Part model, mm, in its own coordinate system. Face numbers are marked on the shaded views. Round coordinates to 2 decimals unless told otherwise and drop trailing zeros. Write each loop counter-clockwise with the first axis right and the second up, starting at its lowest first coordinate (ties: lowest second). Pieces come first, ordered by that corner, then holes. Notation, with made-up numbers: M 34.5,78.25 L 93.5,78.25 A18 cw 93.5,107.25 Z; hole C 48,-16.75 d3. An arc over 180 degrees is marked long. Use a Markdown table: item, result. Add a question column.
1) Two-plate mould, pull along Y, no slides. Class the marked faces 1 and 2: released by +Y, released by -Y, zero draft, split by the parting line, or undercut.
2) Drop flat-ended pins along their axis: P1, Ø3, axis at x = -81.61, y = 42.75, coming from the +Z side (3 decimals); P2, Ø1, axis at y = 17.5, z = 4, coming from the -X side; P3, Ø2.5, axis at x = -2, z = 5, coming from the -Y side; P4, Ø3.5, axis at y = 16, z = 5.5, coming from the +X side. Give the stop position or say it passes through.
3) Slice it at A-A on z = 4.75. Give the number of separate pieces and of enclosed holes in the cut face, plus the area to 3 significant figures.
4) Slice it at C-C on x = -56. Write the cut outline in (y, z) (3 decimals).
5) Wall check: probe 1 along X at (y, z) = (52.5, 4.5) (3 decimals); probe 2 along Y at (x, z) = (-3.5, 3.5) (3 decimals); probe 3 along X at (y, z) = (32, 4.25) (3 decimals). Give the ranges that are in metal, low to high.
6) Slice it at B-B on y = -5. Write the cut outline in (x, z) (3 decimals), plus the area to 3 significant figures.
7) Slice it at D-D on x = 53. Write the cut outline in (y, z) (3 decimals).
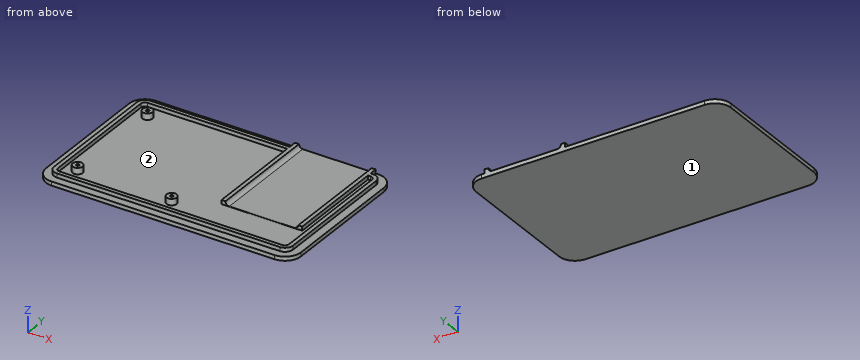
```python
from build123d import *

# Parameters (mm, degrees)
F0_W             = 203.2
F0_H             = 127
F1_DEPTH         = 3.175
F2_R             = 12.7
F4_DEPTH         = 3.175
F5_T             = -3.175
F6_W             = 58
F6_H             = 9.525
F7_DEPTH         = 3.176
F9_DEPTH         = 90
F10_DEPTH        = 3.175
F11_DEPTH        = 3.175
F12_R            = 4
F13_DEPTH        = 5
F17_D            = 2.5
F17_DEPTH        = 5
F17_TIP          = 0.7510757738
F17_ON_F15_D     = 2.5
F17_ON_F15_DEPTH = 5
F17_ON_F15_TIP   = 0.7510757738
F17_ON_F16_D     = 2.5
F17_ON_F16_DEPTH = 5
F17_ON_F16_TIP   = 0.7510757738


# Not quite as in the source:
# - a feature names something its author has since deleted; it is built from what else it names


with BuildPart() as f1:
    # F0 (on Top) → F1 (new body)
    with BuildSketch(Plane.XY):
        Rectangle(F0_W, F0_H)
    extrude(amount=F1_DEPTH)

    # F2
    f2_edges = [f1.edges().sort_by_distance(p)[0] for p in [
        (-101.6, -63.5, 1.5875),
        (-101.6, 63.5, 1.5875),
        (101.6, -63.5, 1.5875),
        (101.6, 63.5, 1.5875),
    ]]
    fillet(f2_edges, radius=F2_R)

    # F3 (on face) → F4 (join)
    with BuildSketch(Plane.XY.offset(3.175)):
        with BuildLine():
            Line((88.9, 57.15), (-88.9, 57.15))
            ThreePointArc((-88.9, 57.15), (-93.3901280605, 55.2901280605), (-95.25, 50.8))
            Line((-95.25, 50.8), (-95.25, -50.8))
            ThreePointArc((-95.25, -50.8), (-93.3901280605, -55.2901280605), (-88.9, -57.15))
            Line((-88.9, -57.15), (88.9, -57.15))
            ThreePointArc((88.9, -57.15), (93.3901280605, -55.2901280605), (95.25, -50.8))
            Line((95.25, -50.8), (95.25, 50.8))
            ThreePointArc((95.25, 50.8), (93.3901280605, 55.2901280605), (88.9, 57.15))
        make_face()
    extrude(amount=F4_DEPTH)

    # F5
    f5_openings = [f1.faces().sort_by_distance(p)[0] for p in [
        (0, 0, 6.35),
    ]]
    offset(amount=F5_T, openings=f5_openings, kind=Kind.INTERSECTION)

    # F6 (on face) → F7 (cut, through all)
    with BuildSketch(Plane.XY.offset(3.175)):
        with Locations((54.6, 58.7375)):
            Rectangle(F6_W, F6_H)
    extrude(amount=F7_DEPTH, mode=Mode.SUBTRACT)

    # F8 (on face) → F9 (join)
    with BuildSketch(Plane(origin=(0, 63.5, 0), x_dir=(-1, 0, 0), z_dir=(0, 1, 0))):
        with BuildLine():
            Line((-83.6, 6.35), (-83.6, 3.175))
            Line((-83.6, 3.175), (-25.6, 3.175))
            Line((-25.6, 3.175), (-25.6, 6.35))
            ThreePointArc((-25.6, 6.35), (-26.4786796564, 4.2286796564), (-28.6, 3.35))
            Line((-28.6, 3.35), (-80.6, 3.35))
            ThreePointArc((-80.6, 3.35), (-82.7213203436, 4.2286796564), (-83.6, 6.35))
        make_face()
    extrude(amount=-F9_DEPTH)

    # F10 (add): faces of the model
    f10_faces = [f1.faces().sort_by_distance(p)[0] for p in [
        (25.6, 13.7375, 4.7625),
        (25.6, 60.325, 4.7625),
    ]]
    extrude(f10_faces, amount=F10_DEPTH)

    # F11 (add): faces of the model
    f11_faces = [f1.faces().sort_by_distance(p)[0] for p in [
        (83.6, 13.7375, 4.7625),
        (83.6, 60.325, 4.7625),
    ]]
    extrude(f11_faces, amount=F11_DEPTH)

    # F12 (on face) → F13 (join)
    with BuildSketch(Plane.XY.offset(3.175)):
        with Locations((-81.6051200401, -42.75)):
            Circle(F12_R)
        with Locations((-6.7051200401, -42.75)):
            Circle(F12_R)
        with Locations((-81.6051200401, 42.75)):
            Circle(F12_R)
    extrude(amount=F13_DEPTH)

    # F17
    with Locations(Plane.XY.offset(8.175)):
        with Locations((-81.6051200401, 42.75)):
            Hole(F17_D / 2, depth=F17_DEPTH)
            with Locations((0, 0, -(F17_DEPTH + F17_TIP / 2))):  # 118° drill point
                Cone(0, F17_D / 2, F17_TIP, mode=Mode.SUBTRACT)

    # F17 on F15
    with Locations(Plane.XY.offset(8.175)):
        with Locations((-81.6051200401, -42.75)):
            Hole(F17_ON_F15_D / 2, depth=F17_ON_F15_DEPTH)
            with Locations((0, 0, -(F17_ON_F15_DEPTH + F17_ON_F15_TIP / 2))):  # 118° drill point
                Cone(0, F17_ON_F15_D / 2, F17_ON_F15_TIP, mode=Mode.SUBTRACT)

    # F17 on F16
    with Locations(Plane.XY.offset(8.175)):
        with Locations((-6.7051200401, -42.75)):
            Hole(F17_ON_F16_D / 2, depth=F17_ON_F16_DEPTH)
            with Locations((0, 0, -(F17_ON_F16_DEPTH + F17_ON_F16_TIP / 2))):  # 118° drill point
                Cone(0, F17_ON_F16_D / 2, F17_ON_F16_TIP, mode=Mode.SUBTRACT)


solid = f1.part
```
Entries:
| question | item | result |
|---|---|---|
| 1 | face 1 | zero draft |
| 1 | face 2 | undercut |
| 2 | P1 | stops at z = 8.175 |
| 2 | P2 | stops at x = -95.25 |
| 2 | P3 | stops at y = -57.15 |
| 2 | P4 | stops at x = 95.25 |
| 3 | separate pieces | 4 |
| 3 | enclosed holes | 3 |
| 3 | area | 2,460 mm^2 |
| 4 | outline | M -63.5,0 L 63.5,0 L 63.5,3.175 L 57.15,3.175 L 57.15,6.35 L 53.975,6.35 L 53.975,3.175 L -53.975,3.175 L -53.975,6.35 L -57.15,6.35 L -57.15,3.175 L -63.5,3.175 Z |
| 5 | probe 1 | x = -95.018 to -91.582, 22.425 to 26.238, 82.962 to 86.775, 91.582 to 95.018 |
| 5 | probe 2 | y = -57.15 to -53.975, -45.143 to -40.357, 53.975 to 57.15 |
| 5 | probe 3 | x = -95.25 to -92.075, 22.425 to 26.458, 82.742 to 86.775, 92.075 to 95.25 |
| 6 | outline | M -101.6,0 L 101.6,0 L 101.6,3.175 L 95.25,3.175 L 95.25,6.35 L 92.075,6.35 L 92.075,3.175 L 86.775,3.175 L 86.775,6.35 L 83.6,6.35 A3 cw 80.6,3.35 L 28.6,3.35 A3 cw 25.6,6.35 L 22.425,6.35 L 22.425,3.175 L -92.075,3.175 L -92.075,6.35 L -95.25,6.35 L -95.25,3.175 L -101.6,3.175 Z |
| 6 | area | 699 mm^2 |
| 7 | outline | M -63.5,0 L 63.5,0 L 63.5,3.35 L -26.5,3.35 L -26.5,3.175 L -53.975,3.175 L -53.975,6.35 L -57.15,6.35 L -57.15,3.175 L -63.5,3.175 Z |
